from build123d import *

# Parameters (mm, degrees)
BOSS_EXTRUDE1_DEPTH = 69.85
SKETCH2_R           = 7.5311
SKETCH2_R_2         = 1.5875
CUT_EXTRUDE1_DEPTH  = 26.4
CUT_EXTRUDE2_DEPTH  = 26.4
CUT_EXTRUDE3_DEPTH  = 26.4


with BuildPart() as part:
    # Sketch1 → Boss-Extrude1 (new body)
    with BuildSketch(Plane(origin=(0, 0, 0), x_dir=(0, 0, -1), z_dir=(1, 0, 0))):
        with BuildLine():
            Line((9.652, 11.176), (-11.176, 11.176))
            Line((-11.176, 11.176), (-12.192, 11.176))
            ThreePointArc((-12.192, 11.176), (-12.551210245, 11.324789755), (-12.7, 11.684))
            Line((-12.7, 11.684), (-12.7, 12.192))
            ThreePointArc((-12.7, 12.192), (-12.551210245, 12.551210245), (-12.192, 12.7))
            Line((-12.192, 12.7), (12.192, 12.7))
            ThreePointArc((12.192, 12.7), (12.551210245, 12.551210245), (12.7, 12.192))
            Line((12.7, 12.192), (12.7, -12.192))
            ThreePointArc((12.7, -12.192), (12.551210245, -12.551210245), (12.192, -12.7))
            Line((12.192, -12.7), (11.684, -12.7))
            ThreePointArc((11.684, -12.7), (11.324789755, -12.551210245), (11.176, -12.192))
            Line((11.176, -12.192), (11.176, -11.176))
            Line((11.176, -11.176), (11.176, 9.652))
            ThreePointArc((11.176, 9.652), (10.729630735, 10.729630735), (9.652, 11.176))
        make_face()
    extrude(amount=BOSS_EXTRUDE1_DEPTH)

    # Sketch2 → Cut-Extrude1 (cut, through all)
    with BuildSketch(Plane(origin=(0, 12.7, 0), x_dir=(1, 0, 0), z_dir=(0, 1, 0))):
        with Locations((17.272, 0)):
            Circle(SKETCH2_R)
        with Locations((29.829368355, 7.25)):
            Circle(SKETCH2_R_2)
        with Locations((4.714631645, -7.25)):
            Circle(SKETCH2_R_2)
    extrude(amount=-CUT_EXTRUDE1_DEPTH, mode=Mode.SUBTRACT)

    # Sketch3 → Cut-Extrude2 (cut, through all)
    with BuildSketch(Plane(origin=(0, 0, -12.7), x_dir=(-1, 0, 0), z_dir=(0, 0, -1))):
        with BuildLine():
            Line((-38.1, 10.084370729), (0, 10.084370729))
            ThreePointArc((0, 10.084370729), (12.7, -2.615629271), (0, -15.315629271))
            Line((0, -15.315629271), (-38.1, -15.315629271))
            Line((-38.1, -15.315629271), (-50.8, -15.315629271))
            Line((-50.8, -15.315629271), (-50.8, -2.615629271))
            ThreePointArc((-50.8, -2.615629271), (-47.080256121, 6.36462685), (-38.1, 10.084370729))
        make_face()
    extrude(amount=-CUT_EXTRUDE2_DEPTH, mode=Mode.SUBTRACT)

    # Sketch4 → Cut-Extrude3 (cut, through all)
    with BuildSketch(Plane(origin=(0, 0, -12.7), x_dir=(-1, 0, 0), z_dir=(0, 0, -1))):
        with BuildLine():
            Line((-65.278, -7.9375), (-65.278, -2.8575))
            ThreePointArc((-65.278, -2.8575), (-63.5, -1.0795), (-61.722, -2.8575))
            Line((-61.722, -2.8575), (-61.722, -7.9375))
            ThreePointArc((-61.722, -7.9375), (-63.5, -9.7155), (-65.278, -7.9375))
        make_face()
        with BuildLine():
            Line((-65.278, 2.8575), (-65.278, 7.9375))
            ThreePointArc((-65.278, 7.9375), (-63.5, 9.7155), (-61.722, 7.9375))
            Line((-61.722, 7.9375), (-61.722, 2.8575))
            ThreePointArc((-61.722, 2.8575), (-63.5, 1.0795), (-65.278, 2.8575))
        make_face()
    extrude(amount=-CUT_EXTRUDE3_DEPTH, mode=Mode.SUBTRACT)


solid = part.part
The listing builds one solid part. Answer for the finished solid, in the listing's coordinates (mm). A direction names the side the tool comes from. Coordinates: 2 decimals unless noted, no trailing zeros. Write each loop counter-clockwise with the first axis right and the second up, starting at its lowest first coordinate (ties: lowest second). Pieces come first, ordered by that corner, then holes. Notation, with made-up numbers: (8, 2) - (12, 2) arc R13 cw to (12, 17) - close; hole circle Ø11 at (72.25, -3.75). An arc over 180 degrees is marked (long way). Put each result on its own line as item: value.
1. The part is cut by section C-C on x = 17.5. Give the vertices of the cut face in (y, z), plus the area to 3 significant figures.
Answer sheet:
outline: (10.08, -12.7) - (12.19, -12.7) arc R0.51 ccw to (12.7, -12.19) - (12.7, -7.53) - (11.18, -7.53) - (11.18, -9.65) arc R1.52 cw to (10.08, -11.11) - close; (11.18, 7.53) - (12.7, 7.53) - (12.7, 12.19) arc R0.51 ccw to (12.19, 12.7) - (11.68, 12.7) arc R0.51 ccw to (11.18, 12.19) - close
area: 17.8 mm^2
2. The part is cut by section D-D on z = 10.5. Give the vertices of the cut face in (x, y), plus the area to 3 significant figures.
Answer sheet:
outline: (0, 11.18) - (69.85, 11.18) - (69.85, 12.7) - (0, 12.7) - close
area: 106 mm^2
3. A tool of negligible diameter and unlimited length cuts with its end or side. For faces 1 (the face through (50.8, -8, -12)), 2 (the face through (63.54, -1.08, -11.95)), 3 (the face through (0, 12, 0)), 4 (the face through (34, 11.176, 1)), from which of +Z, -Z, +X, -X, +Y, -Y can it reach the whole face along a straight path? Write none if from no direction.
Answer sheet:
face 1: +Z, -Z, -X, -Y
face 2: +Z, -Z
face 3: +Z, -Z, -X, +Y, -Y
face 4: +Z, +X, -X, -Y
4. Determine the mould class of faces 5 (the face through (69.85, 5.7, -11.35)), 6 (the face through (34, 12.7, 0)), 7 (the face through (61.722, -5, -12)) for opening direction Y: pulls with the +Y half, pulls with the -Y half, needs draft (parallel to the pull), parting line crosses it, or undercut.
Answer sheet:
face 5: needs draft
face 6: pulls with the +Y half
face 7: undercut
5. The part is cut by section A-A on y = -5. Give the vertices of the cut face in (x, z).
Answer sheet:
outline: (50.8, -12.7) - (61.72, -12.7) - (61.72, -11.18) - (50.8, -11.18) - close; (65.28, -12.7) - (69.85, -12.7) - (69.85, -11.18) - (65.28, -11.18) - close
6. Find the intervals of material crossed by line 1 along Y through (x, z) = (5.5, 10); line 2 along Z through (x, y) = (57, -4); line 3 along Y through (x, z) = (66.5, -10.25), in increasing order. Write a range as from..to.
Answer sheet:
line 1: y = 11.18..12.7
line 2: z = -12.7..-11.18
line 3: y = 11.05..12.7
7. The part is cut by section B-B on z = 0. Give the vertices of the cut face in (x, y).
Answer sheet:
outline: (0, 11.18) - (9.74, 11.18) - (9.74, 12.7) - (0, 12.7) - close; (24.8, 11.18) - (69.85, 11.18) - (69.85, 12.7) - (24.8, 12.7) - close
8. Flat-ended cylindrical pins translate along their axes: pin 1 Ø0.5 at (y, z) = (6.5, -11.5) entering from -X; pin 2 Ø1.7 at (x, z) = (20.5, -12) entering from -Y; pin 3 Ø1.9 at (x, z) = (29.83, -7.25) entering from +Y; pin 4 Ø11 at (x, y) = (55.5, 4) entering from +Z. Find the tip coordinate at first contact, or state that the pin passes through.
Answer sheet:
pin 1: stops at x = 46.68
pin 2: stops at y = 10.08
pin 3: passes through
pin 4: stops at z = -11.18
